Autodesk Inventor part; units mm, degrees
ref_plane "YZ Plane" through (0, 0, 0) normal (1, 0, 0) x (0, 1, 0)
ref_plane "XZ Plane" through (0, 0, 0) normal (0, 1, 0) x (-1, 0, 0)
ref_plane "XY Plane" through (0, 0, 0) normal (0, 0, 1) x (1, 0, 0)
sketch "Sketch1" plane through (0, 0, 0) normal (0, 0, 1) x (1, 0, 0)
  line L0 (15.2998, 26.5) -> (15.2998, -26.5) construction
  line L1 (15.2998, -26.5) -> (-30.5996, 0) construction
  line L2 (-30.5996, 0) -> (15.2998, 26.5) construction
  line L3 (0, 48.0119) -> (0, -48.0119)
  circle A0 centre (0, 0) radius 12.5
  line L4 (24.9, -24.45) -> (-24.9, -24.45) construction
  line L5 (-24.9, -24.45) -> (-24.9, 24.45) construction
  line L6 (-24.9, 24.45) -> (24.9, 24.45) construction
  line L7 (24.9, 24.45) -> (24.9, -24.45) construction
  line L8 (24.9, -24.45) -> (-24.9, 24.45) construction
  line L9 (-24.9, -24.45) -> (24.9, 24.45) construction
  line L10 (20, -20) -> (-20, -20) construction
  line L11 (-20, -20) -> (-20, 20) construction
  line L12 (-20, 20) -> (20, 20) construction
  line L13 (20, 20) -> (20, -20) construction
  line L14 (20, -20) -> (-20, 20) construction
  line L15 (-20, -20) -> (20, 20) construction
  line L16 (-37.5996, -1.7321) -> (17.2998, -33.4282)
  line L17 (20.2998, -31.6962) -> (20.2998, 31.6962)
  line L18 (17.2998, 33.4282) -> (-37.5996, 1.7321)
  arc A1 (-37.5996, 1.7321) -> (-37.5996, -1.7321) centre (-36.5996, 0) ccw
  arc A2 (20.2998, 31.6962) -> (17.2998, 33.4282) centre (18.2998, 31.6962) ccw
  arc A3 (17.2998, -33.4282) -> (20.2998, -31.6962) centre (18.2998, -31.6962) ccw
  circle A4 centre (15.2998, 26.5) radius 2
  circle A5 centre (-30.5996, 0) radius 2
  circle A6 centre (15.2998, -26.5) radius 2
  dimension "d1" = 53
  dimension "d2" = 25
  dimension "d3" = 49.8
  dimension "d4" = 48.9
  dimension "d5" = 40
  dimension "d6" = 40
  dimension "d7" = 5
  dimension "d8" = 2
  dimension "d9" = 4
  dimension "d10" = 4
  dimension "d11" = 4
extrude "Extrusion1" add sketch "Sketch1" along normal blind 3 contours L18 A2 L17 A3 L16 L3 A0 | L3 A0 L16 A1 L18
sketch "Sketch3" plane through (0, 0, 3) normal (0, 0, 1) x (1, 0, 0)
  circle A0 centre (0, 0) radius 12.5
  circle A1 centre (15.2998, -26.5) radius 2
  circle A2 centre (-30.5996, 0) radius 2
  circle A3 centre (15.2998, 26.5) radius 2
  line L0 (-37.5996, -1.7321) -> (17.2998, -33.4282)
  arc A4 (17.2998, -33.4282) -> (20.2998, -31.6962) centre (18.2998, -31.6962) ccw
  line L1 (20.2998, -31.6962) -> (20.2998, 31.6962)
  arc A5 (20.2998, 31.6962) -> (17.2998, 33.4282) centre (18.2998, 31.6962) ccw
  line L2 (17.2998, 33.4282) -> (-37.5996, 1.7321)
  arc A6 (-37.5996, 1.7321) -> (-37.5996, -1.7321) centre (-36.5996, 0) ccw
  line L3 (22, -24) -> (-22, -24)
  line L4 (-24, -22) -> (-24, 22)
  line L5 (-22, 24) -> (22, 24)
  line L6 (24, 22) -> (24, -22)
  line L7 (24, -24) -> (-24, 24) construction
  line L8 (-24, -24) -> (24, 24) construction
  arc A7 (-22, 24) -> (-24, 22) centre (-22, 22) ccw
  arc A8 (-24, -22) -> (-22, -24) centre (-22, -22) ccw
  arc A9 (22, -24) -> (24, -22) centre (22, -22) ccw
  arc A10 (24, 22) -> (22, 24) centre (22, 22) ccw
  line L9 (17.2998, 33.4282) -> (-37.5996, 1.7321)
  line L10 (-37.5996, -1.7321) -> (17.2998, -33.4282)
  line L11 (20.2998, -31.6962) -> (20.2998, 31.6962)
  point P0 (20.2998, 24)
  point P1 (-24, 9.5838)
  point P2 (-24, -9.5838)
  point P3 (0.9697, -24)
  point P4 (20.2998, -24)
  dimension "d14" = 48
  dimension "d15" = 48
  dimension "d16" = 2
extrude "Extrusion2" add sketch "Sketch3" along normal blind 5 contours A0 | A1 | A3 | A6 L2 L4 L0 | L4 L2 L5 L1 L3 L0 | L0 L3 A8 L4 | L3 L1 A4 L0 | L4 A7 L5 L2 | L1 L5 A10 L6 A9 L3 | L2 A5 L1 L5
sketch "Sketch4" plane through (0, 0, 8) normal (0, 0, 1) x (1, 0, 0)
  circle A0 centre (0, 0) radius 12.5
  line L0 (20, -20) -> (-20, -20) construction
  line L1 (-20, -20) -> (-20, 20) construction
  line L2 (-20, 20) -> (20, 20) construction
  line L3 (20, 20) -> (20, -20) construction
  line L4 (20, -20) -> (-20, 20) construction
  line L5 (-20, -20) -> (20, 20) construction
  circle A1 centre (15.2998, 26.5) radius 2
  circle A2 centre (15.2998, -26.5) radius 2
  dimension "d19" = 40
  dimension "d20" = 40
extrude "Extrusion3" cut sketch "Sketch4" against normal through all
ref_plane "Work Plane1" through (-22, 0, 3) normal (0, 1, 0) x (1, 0, 0)
ref_plane "Work Plane2" through (0, -22, 3) normal (-1, 0, 0) x (0, 0, 1)
ref_plane "Work Plane3" through (-22, -20, 3) normal (0, 1, 0) x (1, 0, 0)
sketch "Sketch5" plane through (-22, -20, 3) normal (0, 1, 0) x (1, 0, 0)
  line L0 (22.9697, 0) -> (22.9697, -5)
  line L1 (22.9697, 0) -> (0, 0)
  line L2 (0, 0) -> (0, -5)
  line L3 (22.9697, -5) -> (0, -5)
  circle A0 centre (2, -4.2) radius 2.5
  line L4 (22, -11.7547) -> (22, 5.4591)
  line L5 (-0.5, -4.2) -> (4.5, -4.2)
  line L6 (0, 0) -> (0, -5)
  point P0 (22, 3)
  dimension "d24" = 5
  dimension "d25" = 20
  dimension "d26" = 0.8
revolve "Revolution1" cut sketch "Sketch5" angle 360 about axis through (-22.5, -20, 7.2) along (1, 0, 0) contours A0 L5 L2 L3 | L3 L2 L5 A0
pattern_linear "Rectangular Pattern1" count 2 spacing 40 along (1, 0, 0) count 2 spacing 40 along (0, 1, 0) of "Revolution1"
properties part number "20_Cube_Insert_Openflexure_Deltastage_Adapter"
Build history of the part. All positions in model axes, mm. A direction names the side the tool comes from. Round coordinates to 2 decimals unless told otherwise and drop trailing zeros. Order: outer loops, then holes, each group sorted by start corner. A loop starts at its lowest first (then second) coordinate and runs counter-clockwise, first axis right, second up. Notation, with made-up numbers: M -23,60 L 30,60 A14 cw 30,72 Z; hole C 80,-6.75 d3. An arc over 180 degrees is marked long. Use CSV: the item, a comma, the result in double quotes. Start each with the question number.
(1) Cut at A-A on y = 0. List the corners of the cut face in (x, z), then the cut area to 3 significant figures.
(2) Cut at C-C on z = 2. List the corners of the cut face in (x, y), then the cut area to 3 significant figures.
(3) Drill centre lines: probe 1 along X at (y, z) = (-1, 1); probe 2 along Y at (x, z) = (-21.5, 7.25); probe 3 along Z at (x, y) = (-13.5, 20). Where is each one in solid material? Low to high.
(4) Tool access for faces 4 (the face through (-11, 24, 5)), 5 (the face through (-14, 18, 3)), 6 (the face through (21, -24, 5)): list every direction of +Z, -Z, +X, -X, +Y, -Y with a clear straight run to the whole face (end or side of a thin tool).
(5) Cut at D-D on z = 5.75. State how many separate pieces and enclosed holes the cut face has, then the cut area to 3 significant figures.
(6) Mould opens along X. For faces 1 (the face through (-1, 13, 0)), 2 (the face through (13.7, 25.3, 4.1)), 3 (the face through (19.33, -33.41, 3.94)) say: +X half, -X half, draft (parallel to the pull), parting line (faces both ways), or undercut.
(7) Flat gauge pins, fed straight in: P1, Ø4, axis at y = 16.5, z = 6, coming from the -X side; P2, Ø4, axis at x = -13, z = 6, coming from the -Y side; P3, Ø1.9, axis at x = 21, z = 5, coming from the -Y side. Where does each tip first touch, or does it go through?
(8) Cut at B-B on x = 5.5. List the corners of the cut face in (y, z).
Findings:
1,outline,"M -38.6,0 L -32.6,0 L -32.6,8 L -38.6,8 Z; M -28.6,0 L -12.5,0 L -12.5,8 L -28.6,8 Z; M 12.5,0 L 20.3,0 L 20.3,3 L 24,3 L 24,8 L 12.5,8 Z"
1,area,"258 mm^2"
2,outline,"M -37.6,-1.73 L 17.3,-33.43 A2 ccw 20.3,-31.7 L 20.3,31.7 A2 ccw 17.3,33.43 L -37.6,1.73 A2 ccw Z; hole C -30.6,0 d4; hole C 0,0 d25; hole C 15.3,-26.5 d4; hole C 15.3,26.5 d4"
2,area,"1,600 mm^2"
3,probe 1,"x = -38.33 to -32.33, -28.87 to -12.46, 12.46 to 20.3"
3,probe 2,"y = -24 to -22, -18 to 18, 22 to 24"
3,probe 3,"z = 3 to 8"
4,face 4,"+Z, -Z, -X, +Y"
4,face 5,"-Z, -X, +Y"
4,face 6,"+Z, -Z, +X, -Y"
5,separate pieces,"1"
5,enclosed holes,"8"
5,area,"2,090 mm^2"
6,face 1,"draft"
6,face 2,"undercut"
6,face 3,"parting line"
7,P1,"stops at x = -24"
7,P2,"stops at y = -24"
7,P3,"stops at y = -32.66"
8,outline,"M -26.62,0 L -11.22,0 L -11.22,8 L -26.62,8 Z; M 11.22,0 L 26.62,0 L 26.62,8 L 11.22,8 Z"
